from build123d import *

# Parameters (mm, degrees)
F0_W          = 11
F0_H          = 4
F1_DEPTH      = 6
F1_DEPTH_BACK = 6
F2_R          = 5.5
F2_R_2        = 2.4
F3_DEPTH      = 4
F4_DEPTH      = 10.8
F5_R          = 2.4
F6_DEPTH      = 4
F7_DEPTH      = 10
F8_R          = 2.3
F9_DEPTH      = 3
F10_DEPTH     = 14


# Not quite as in the source:
# - a feature names something its author has since deleted; it is built from what else it names


with BuildPart() as f1:
    # F0 (on Top) → F1 (new body, two sides)
    with BuildSketch(Plane.XY) as f1_sk:
        with Locations((0, 37)):
            Rectangle(F0_W, F0_H)
        with BuildLine():
            ThreePointArc((-9.5, 35), (-8.6213203436, 32.8786796564), (-6.5, 32))
            Line((-6.5, 32), (5.8594679956, 32))
            ThreePointArc((5.8594679956, 32), (23.5324507486, 25.5063318649), (34.5083337044, 10.2082261463))
            Line((34.5083337044, 10.2082261463), (34.5083337044, -10.2082261463))
            ThreePointArc((34.5083337044, -10.2082261463), (23.5324507486, -25.5063318649), (5.8594679956, -32))
            Line((5.8594679956, -32), (-6.5, -32))
            ThreePointArc((-6.5, -32), (-8.6213203436, -32.8786796564), (-9.5, -35))
            Line((-9.5, -35), (-9.5, -39))
            Line((-9.5, -39), (-5.5, -39))
            Line((-5.5, -39), (-5.5, -35))
            Line((-5.5, -35), (5.5, -35))
            Line((5.5, -35), (5.5, -39))
            ThreePointArc((5.5, -39), (27.2702801405, -28.8873683489), (39.0994077402, -8))
            Line((39.0994077402, -8), (40.2236692607, -8))
            Line((40.2236692607, -8), (40.2236692607, 8))
            Line((40.2236692607, 8), (39.0994077402, 8))
            ThreePointArc((39.0994077402, 8), (27.2702801405, 28.8873683489), (5.5, 39))
            Line((5.5, 39), (5.5, 35))
            Line((5.5, 35), (-5.5, 35))
            Line((-5.5, 35), (-5.5, 39))
            Line((-5.5, 39), (-9.5, 39))
            Line((-9.5, 39), (-9.5, 35))
        make_face()
        with Locations((0, -37)):
            Rectangle(F0_W, F0_H)
    extrude(amount=F1_DEPTH)
    extrude(f1_sk.sketch, amount=-F1_DEPTH_BACK)

    # F2 (on face) → F3 (cut)
    with BuildSketch(Plane.XZ.offset(39)):
        Circle(F2_R)
        Circle(F2_R_2, mode=Mode.SUBTRACT)
    extrude(amount=-F3_DEPTH, mode=Mode.SUBTRACT)

    # F4 (cut): a face of the model
    f4_faces = [f1.faces().sort_by_distance(p)[0] for p in [
        (0, -39, 0),
    ]]
    extrude(f4_faces, amount=-F4_DEPTH, mode=Mode.SUBTRACT)

    # F5 (on face) → F6 (cut)
    with BuildSketch(Plane(origin=(0, 39, 0), x_dir=(-1, 0, 0), z_dir=(0, 1, 0))):
        with BuildLine():
            ThreePointArc((-5.5, 3.96e-08), (-1.98e-08, -5.5), (5.5, 0))
            ThreePointArc((5.5, 0), (1.98e-08, 5.5), (-5.5, 3.96e-08))
        make_face()
        Circle(F5_R, mode=Mode.SUBTRACT)
    extrude(amount=-F6_DEPTH, mode=Mode.SUBTRACT)

    # F7 (cut): a face of the model
    f7_faces = [f1.faces().sort_by_distance(p)[0] for p in [
        (0, 39, 0),
    ]]
    extrude(f7_faces, amount=-F7_DEPTH, mode=Mode.SUBTRACT)

    # F8 (on face) → F9 (cut)
    with BuildSketch(Plane.YZ.offset(40.2236692607)):
        Polygon((2.7135462652, -4.7), (5.4270925304, 0), (2.7135462652, 4.7), (-2.7135462652, 4.7), (-5.4270925304, 0), (-2.7135462652, -4.7), align=None)
        Circle(F8_R, mode=Mode.SUBTRACT)
    extrude(amount=-F9_DEPTH, mode=Mode.SUBTRACT)

    # F10 (cut): a face of the model
    f10_faces = [f1.faces().sort_by_distance(p)[0] for p in [
        (40.2236692607, 0, 0),
    ]]
    extrude(f10_faces, amount=-F10_DEPTH, mode=Mode.SUBTRACT)


solid = f1.part
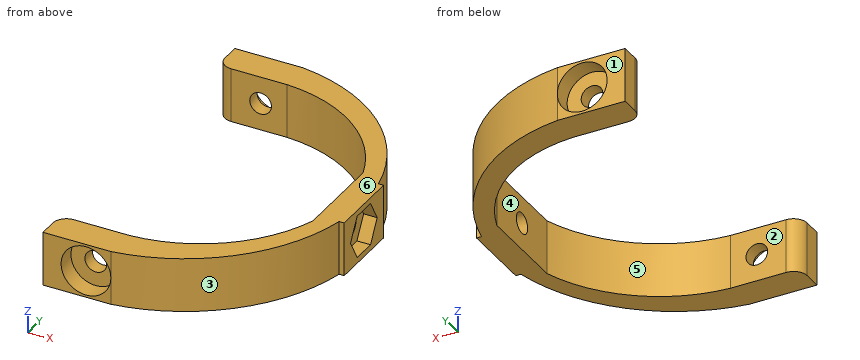
Input: part model. Units: mm. Frame: model coordinates. Face numbers are marked on the shaded views. A direction names the side the tool comes from. Coordinates: 2 decimals unless noted, no trailing zeros. Loops run counter-clockwise (first coordinate to the right, second up) from the corner with the lowest first, then second, coordinate; pieces in that order, holes last.
(1) Section B-B on x = 0. Return the cut outline in (y, z), then the cut area to 3 significant figures.
(2) Section A-A on y = 0. Return the cut outline in (x, z), then the cut area to 3 significant figures.
(3) Section D-D on z = -1.25. Count the separate pieces of the cut face and the enclosed holes in it, then the cut area to 3 significant figures.
(4) Material intervals for probe 1 along Z at (x, y) = (0, 37.15); probe 2 along Z at (x, y) = (0, 34); probe 3 along Y at (x, z) = (-6, -1), sorted ascending.
(5) First-contact query: pin 1 Ø4 at (x, z) = (8.5, 3) entering from +Y; pin 2 Ø3.5 at (x, z) = (2, 1.5) entering from +Y; pin 3 Ø3 at (x, z) = (34.5, 2) entering from -Y. Flat tips, straight axial feed; report the tip coordinate or a pass-through.
(6) Pull-direction query (Y, two-part tool) for the marked faces 3, 4, 5 and 6; classes: released by +Y, released by -Y, zero draft, split by the parting line, or undercut.
(7) Set-up query: the marked faces 1 and 2. Return all of +Z, -Z, +X, -X, +Y, -Y with unobstructed straight access to the full face (end or side cutting, diameter ignored); none if empty.
(8) Section C-C on x = 32.5. Return the cut outline in (y, z), then the cut area to 3 significant figures.
Data:
1. outline: (-39, -6) - (-32, -6) - (-32, -2.4) - (-35, -2.4) - (-35, -5.5) - (-39, -5.5) - close; (-39, 5.5) - (-35, 5.5) - (-35, 2.4) - (-32, 2.4) - (-32, 6) - (-39, 6) - close; (32, -6) - (39, -6) - (39, -5.5) - (35, -5.5) - (35, -2.4) - (32, -2.4) - close; (32, 2.4) - (35, 2.4) - (35, 5.5) - (39, 5.5) - (39, 6) - (32, 6) - close
1. area: 51.2 mm2
2. outline: (34.51, -6) - (40.22, -6) - (40.22, -4.7) - (37.22, -4.7) - (37.22, -2.3) - (34.51, -2.3) - close; (34.51, 2.3) - (37.22, 2.3) - (37.22, 4.7) - (40.22, 4.7) - (40.22, 6) - (34.51, 6) - close
2. area: 27.9 mm2
3. separate pieces: 4
3. enclosed holes: 0
3. area: 608 mm2
4. probe 1: z = -6 to -5.5, 5.5 to 6
4. probe 2: z = -6 to -2.4, 2.4 to 6
4. probe 3: y = -39 to -32, 32 to 39
5. pin 1: stops at y = 38.86
5. pin 2: stops at y = 35
5. pin 3: stops at y = -22.28
6. face 3: released by -Y
6. face 4: undercut
6. face 5: undercut
6. face 6: zero draft
7. face 1: +Z, -Z, +X, -X, +Y
7. face 2: +Z, -Z, -X
8. outline: (-22.99, -6) - (-14.91, -6) - (-14.91, 6) - (-22.99, 6) - close; (14.91, -6) - (22.99, -6) - (22.99, 6) - (14.91, 6) - close
8. area: 194 mm2
